from build123d import *

# Parameters (mm, degrees)
F4_W     = 100
F4_H     = 65
F0_DEPTH = 5
F2_DEPTH = 5.001
F5_D     = 5


with BuildPart() as f0:
    # F4 (on Top) → F0 (new body)
    with BuildSketch(Plane.XY):
        Rectangle(F4_W, F4_H)
    extrude(amount=F0_DEPTH)

    # F1 (on face) → F2 (cut, through all)
    with BuildSketch(Plane.XY.offset(5)):
        with BuildLine():
            ThreePointArc((50, -30), (71.2132034356, -21.2132034356), (80, 0))
            ThreePointArc((80, 0), (71.2132034356, 21.2132034356), (50, 30))
            Line((50, 30), (50, -30))
        make_face()
        with BuildLine():
            Line((50, -30), (50, 30))
            ThreePointArc((50, 30), (20, 0), (50, -30))
        make_face()
    extrude(amount=-F2_DEPTH, mode=Mode.SUBTRACT)

    # F5 (through all)
    with Locations(Plane.XY.offset(5)):
        with Locations((-30, 17.5), (-30, -17.5)):
            Hole(F5_D / 2)


solid = f0.part
Model file for the job. Use its own axes, mm. Give positions to 0.01 mm unless a question says otherwise; leave off trailing zeros. Write each loop counter-clockwise with the first axis right and the second up, starting at its lowest first coordinate (ties: lowest second). Pieces come first, ordered by that corner, then holes. Notation, with made-up numbers: M 89.25,35 L 111.25,35 A28 cw 111.25,74 Z; hole C 15,76 d4. An arc over 180 degrees is marked long. One line per item, written item: value. Start each with the question number.
Q1. Saw through at A-A, the plane x = -30. Write the cut outline in (y, z).
Q2. Two-plate mould, pull along Y, no slides. Class faces 1 (the flat face through (-50, 0, 2)), 2 (the flat face through (-1, 32.5, 2)), 3 (the cylindrical face through (-28, -19, 2)): +Y half, -Y half, draft (parallel to the pull), parting line (faces both ways), or undercut.
Q3. Drop a flat-ended pin along its axis: pin 1 Ø6 at (x, y) = (-30, 17.5) entering from +Z. Give the stop position or say it passes through.
Q4. Probe probe 1 along Y at (x, z) = (-30, 3.4); probe 2 along Y at (x, z) = (-32, 4); probe 3 along X at (y, z) = (-0.5, 0.4). List the from-to ranges inside material, lowest first. Write a range as [from, to].
Q5. Saw through at B-B, the plane y = 17.5. Write the cut outline in (x, z).
Q6. Saw through at C-C, the plane z = 2.95. Write the cut outline in (x, y).
Q7. Saw through at D-D, the plane x = 21. Write the cut outline in (y, z), plus the area to 3 significant figures.
Output values:
1. outline: M -32.5,0 L -20,0 L -20,5 L -32.5,5 Z; M -15,0 L 15,0 L 15,5 L -15,5 Z; M 20,0 L 32.5,0 L 32.5,5 L 20,5 Z
2. face 1: draft
2. face 2: +Y half
2. face 3: undercut
3. pin 1: stops at z = 5
4. probe 1: y = [-32.5, -20], [-15, 15], [20, 32.5]
4. probe 2: y = [-32.5, -19], [-16, 16], [19, 32.5]
4. probe 3: x = [-50, 20]
5. outline: M -50,0 L -32.5,0 L -32.5,5 L -50,5 Z; M -27.5,0 L 25.63,0 L 25.63,5 L -27.5,5 Z
6. outline: M -50,-32.5 L 50,-32.5 L 50,-30 A30 cw 50,30 L 50,32.5 L -50,32.5 Z; hole C -30,-17.5 d5; hole C -30,17.5 d5
7. outline: M -32.5,0 L -7.68,0 L -7.68,5 L -32.5,5 Z; M 7.68,0 L 32.5,0 L 32.5,5 L 7.68,5 Z
7. area: 248 mm²
